```python
from build123d import *

# Parameters (mm, degrees)
SKETCH1_W           = 300
SKETCH1_H           = 240
BOSS_EXTRUDE1_DEPTH = 5
SKETCH2_R           = 10.25
SKETCH2_R_2         = 11.58
SKETCH2_R_3         = 3.4
SKETCH2_R_4         = 3.1
SKETCH2_R_5         = 1.5
SKETCH2_W           = 60
SKETCH2_H           = 30
CUT_EXTRUDE4_DEPTH  = 193.158788506


with BuildPart() as part:
    # Sketch1 → Boss-Extrude1 (new body)
    with BuildSketch(Plane(origin=(0, 0, 0), x_dir=(1, 0, 0), z_dir=(0, 1, 0))):
        Rectangle(SKETCH1_W, SKETCH1_H)
    extrude(amount=BOSS_EXTRUDE1_DEPTH)

    # Sketch2 → Cut-Extrude4 (cut, through all)
    with BuildSketch(Plane(origin=(0, 0, 0), x_dir=(1, 0, 0), z_dir=(0, 1, 0))):
        with Locations(Location((-96.25, 80, 0), (0, 0, 270))):
            Circle(SKETCH2_R)
        with Locations(Location((-96.25, -40, 0), (0, 0, 270))):
            Circle(SKETCH2_R_2)
        with Locations(Location((-96.25, -80, 0), (0, 0, 270))):
            Circle(SKETCH2_R_2)
        with Locations(Location((-96.25, 40, 0), (0, 0, 270))):
            Circle(SKETCH2_R_3)
        with Locations(Location((-32.08, -60, 0), (0, 0, 270))):
            Circle(SKETCH2_R_2)
        with Locations(Location((32.08, -60, 0), (0, 0, 270))):
            Circle(SKETCH2_R_2)
        with Locations(Location((96.25, -60, 0), (0, 0, 270))):
            Circle(SKETCH2_R_4)
        with Locations(Location((36.5, 38.5, 0), (0, 0, 270))):
            Circle(SKETCH2_R_5)
        with Locations(Location((36.5, 81.5, 0), (0, 0, 270))):
            Circle(SKETCH2_R_5)
        with Locations(Location((-36.5, 81.5, 0), (0, 0, 270))):
            Circle(SKETCH2_R_5)
        with Locations(Location((-36.5, 38.5, 0), (0, 0, 270))):
            Circle(SKETCH2_R_5)
        with Locations((0, 60)):
            Rectangle(SKETCH2_W, SKETCH2_H)
    extrude(amount=CUT_EXTRUDE4_DEPTH, mode=Mode.SUBTRACT)


solid = part.part
```
Here's how the part is built. I have some questions about the finished solid (model axes, mm). Round coordinates to 2 decimals unless told otherwise and drop trailing zeros. Loops run counter-clockwise (first coordinate to the right, second up) from the corner with the lowest first, then second, coordinate; pieces in that order, holes last. Notation, with made-up numbers: (86.25, 40) -> (126.25, 40) arc R26 cw to (126.25, 62) -> close; hole circle Ø10 at (-34, -13.5). An arc over 180 degrees is marked (long way). Answer as CSV lines item,"result".
1. Thinking about a two-plate mould opening in Z: for faces 1 (the face through (-2, 5, -2)), 2 (the face through (-28.602, 2.465, 71.045)), which applies, released by +Z, released by -Z, zero draft, split by the parting line, or undercut?
Final values:
face 1,"zero draft"
face 2,"undercut"
2. If we section it at B-B on x = 0: Please give me the cut outline in (y, z).
Final values:
outline,"(0, -120) -> (5, -120) -> (5, -75) -> (0, -75) -> close; (0, -45) -> (5, -45) -> (5, 120) -> (0, 120) -> close"
3. If I drill on L1, parallel to X at y = 2, z = 60; L2, parallel to Z at x = -96.25, y = 3.5; L3, parallel to X at y = 4.5, z = 50, over which ranges is the centre line in solid material (lowest first)?
Final values:
L1,"x = -150 to -43.66, -20.5 to 20.5, 43.66 to 93.15, 99.35 to 150"
L2,"z = -120 to -90.25, -69.75 to -43.4, -36.6 to 28.42, 51.58 to 68.42, 91.58 to 120"
L3,"x = -150 to -102.09, -90.41 to -37.92, -26.24 to 26.24, 37.92 to 150"
4. If we section it at C-C on y = 3.8: Count the separate pieces of the cut face and the enclosed holes in it, plus the area to 3 significant figures.
Final values:
separate pieces,"1"
enclosed holes,"12"
area,"68,100 mm^2"
5. If we section it at A-A on z = -56.5: Please give me the cut outline in (x, y).
Final values:
outline,"(-150, 0) -> (-30, 0) -> (-30, 5) -> (-150, 5) -> close; (30, 0) -> (150, 0) -> (150, 5) -> (30, 5) -> close"
